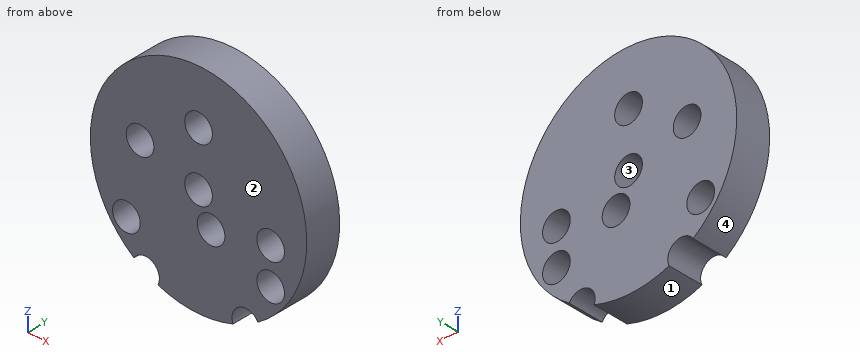
```python
from build123d import *

# Parameters (mm, degrees)
SKETCH1_R              = 76.2
BOSS_EXTRUDE1_DEPTH    = 25.4
M22X2_5_TAPPED_HOLE1_D = 19.5


with BuildPart() as part:
    # Sketch1 → Boss-Extrude1 (new body)
    with BuildSketch(Plane(origin=(0, 0, 0), x_dir=(1, 0, 0), z_dir=(0, 1, 0))):
        with Locations(Location((0, 0, 0), (0, 0, 270))):
            Circle(SKETCH1_R)
    extrude(amount=-BOSS_EXTRUDE1_DEPTH)

    # M22x2.5 Tapped Hole1 (through all)
    with Locations(Plane(origin=(0, 0, 0), x_dir=(1, 0, 0), z_dir=(0, 1, 0))):
        with Locations((50.8, 12.7), (0, -38.1), (0, 0), (-50.8, 38.1), (50.8, 38.1), (-37.337291981, 66.425647362), (33.306888382, 68.535328016), (8.79976324, 20.818952057), (-41.20864737, -12.877702303)):
            Hole(M22X2_5_TAPPED_HOLE1_D / 2)


solid = part.part
```
Input: part model. Units: mm. Frame: model coordinates. Face numbers are marked on the shaded views. Round coordinates to 2 decimals unless told otherwise and drop trailing zeros. Loops run counter-clockwise (first coordinate to the right, second up) from the corner with the lowest first, then second, coordinate; pieces in that order, holes last.
1) Section query D-D on y = -12.25. Return the cut outline in (x, z).
Ans:
outline: (-45.51, -61.11) arc R9.75 cw to (-28.55, -70.65) arc R76.2 ccw to (24.28, -72.23) arc R9.75 cw to (41.79, -63.72) arc R76.2 ccw (long way) to start; hole circle Ø19.5 at (-50.8, -38.1); hole circle Ø19.5 at (-41.21, 12.88); hole circle Ø19.5 at (0, 0); hole circle Ø19.5 at (0, 38.1); hole circle Ø19.5 at (8.8, -20.82); hole circle Ø19.5 at (50.8, -38.1); hole circle Ø19.5 at (50.8, -12.7)
2) Pin query (flat end, axial travel): pin 1 (3 mm diameter, centred on y = -12.5, z = 33.5, fed in from +X); pin 2 (1 mm diameter, centred on y = -19, z = 34.5, fed in from +X); pin 3 (10 mm diameter, centred on x = -19, y = -7.5, fed in from -Z). Return the tip coordinate at first contact, or that it passes through.
Ans:
pin 1: stops at x = 69.16
pin 2: stops at x = 68.19
pin 3: stops at z = -74.9
3) Pull-direction query (Z, two-part tool) for the marked faces 1, 2, 3 and 4; classes: released by +Z, released by -Z, zero draft, split by the parting line, or undercut.
Ans:
face 1: released by -Z
face 2: zero draft
face 3: undercut
face 4: split by the parting line
4) Section query B-B on x = -4.5. Return the cut outline in (y, z), plus the area to 3 significant figures.
Ans:
outline: (-25.4, -76.07) - (0, -76.07) - (0, -8.65) - (-25.4, -8.65) - close; (-25.4, 8.65) - (0, 8.65) - (0, 29.45) - (-25.4, 29.45) - close; (-25.4, 46.75) - (0, 46.75) - (0, 76.07) - (-25.4, 76.07) - close
area: 2,990 mm2
5) Section query A-A on z = 0. Return the cut outline in (x, y).
Ans:
outline: (-76.2, -25.4) - (-9.75, -25.4) - (-9.75, 0) - (-76.2, 0) - close; (9.75, -25.4) - (76.2, -25.4) - (76.2, 0) - (9.75, 0) - close
6) Section query C-C on z = -38.1. Return the cut outline in (x, y), plus the area to 3 significant figures.
Ans:
outline: (-65.99, -25.4) - (-60.55, -25.4) - (-60.55, 0) - (-65.99, 0) - close; (-41.05, -25.4) - (41.05, -25.4) - (41.05, 0) - (-41.05, 0) - close; (60.55, -25.4) - (65.99, -25.4) - (65.99, 0) - (60.55, 0) - close
area: 2,360 mm2
7) Material intervals for line 1 (Z direction, x = 0, y = -7.5); line 2 (X direction, y = -5.5, z = -20); line 3 (Z direction, x = 4.5, y = -19), sorted ascending.
Ans:
line 1: z = -76.2 to -25.02, -16.62 to -9.75, 9.75 to 28.35, 47.85 to 76.2
line 2: x = -73.53 to -0.92, 18.52 to 44.34, 57.26 to 73.53
line 3: z = -76.07 to -29.57, -12.07 to -8.65, 8.65 to 29.45, 46.75 to 76.07
